The model under review builds one solid part; all positions refer to its coordinate system, in mm. Face numbers are marked on the shaded views. Round coordinates to 2 decimals unless told otherwise and drop trailing zeros. Order: outer loops, then holes, each group sorted by start corner. A loop starts at its lowest first (then second) coordinate and runs counter-clockwise, first axis right, second up. Notation, with made-up numbers: M 89,36.25 L 143,36.25 A20 ccw 143,49.25 Z; hole C -16.5,-33.5 d10. An arc over 180 degrees is marked long. Answer as a JSON object with one key per item and string values. Group by question number.
1) Consider section B-B, the plane z = -2.5. Write out the cut boundary in (x, y).
2) The part is to be moulded in two halves that separate along X. For the marked faces 1 and 2, say which applies: +X half, -X half, draft (parallel to the pull), parting line (faces both ways), or undercut.
3) Consider section A-A, the plane x = 5. Write out the cut boundary in (y, z), then the cut area to 3 significant figures.
4) To check wall thickness, follow line 1 (Y direction, x = -85, z = 0.1); line 2 (X direction, y = 121.75, z = 0.4); line 3 (X direction, y = 29, z = -4.75). State the ranges of each line that lie inside material, in increasing order.
5) Insertion check: pin 1 Ø6 at (x, y) = (5.5, 46.5) entering from -Z; pin 2 Ø3 at (x, y) = (5, 31.75) entering from -Z; pin 3 Ø3.5 at (y, z) = (56, -2) entering from -X; pin 4 Ø1 at (y, z) = (90.5, -2) entering from +X. Each pin has a flat end and moves straight along its axis. Give the tip position at first contact, or say it passes through.
6) Consider section D-D, the plane y = 89.5. Write out the cut boundary in (x, z), then the cut area to 3 significant figures.
7) Consider section C-C, the plane y = 121.75. Write out the cut boundary in (x, z).
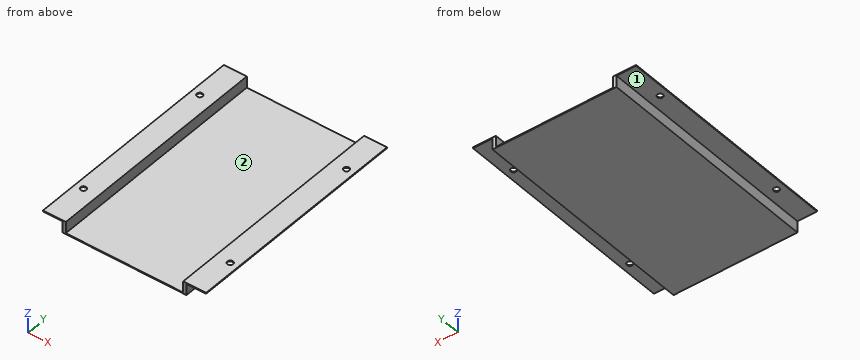
Autodesk Inventor part; units mm, degrees
ref_plane "YZ Plane" through (0, 0, 0) normal (1, 0, 0) x (0, 1, 0)
ref_plane "XZ Plane" through (0, 0, 0) normal (0, 1, 0) x (-1, 0, 0)
ref_plane "XY Plane" through (0, 0, 0) normal (0, 0, 1) x (1, 0, 0)
sketch "Skizze1" plane through (0, 0, 0) normal (0, 0, 1) x (1, 0, 0)
  line L0 (-90, 0) -> (-90, 36.75) construction
  line L1 (10, 0) -> (10, 36.75) construction
  line L2 (-90, 116.75) -> (-90, 147.085) construction
  line L3 (10, 147.085) -> (10, 116.75) construction
  circle A0 centre (-85, 121.75) radius 1.75
  circle A1 centre (5, 121.75) radius 1.75
  circle A2 centre (-85, 31.75) radius 1.75
  circle A3 centre (5, 31.75) radius 1.75
  line L4 (-90, 6.75) -> (10, 6.75)
  line L5 (10, 6.75) -> (10, 146.75)
  line L6 (10, 146.75) -> (-90, 146.75)
  line L7 (-90, 146.75) -> (-90, 6.75)
  point P0 (0, 0)
  dimension "d0" = 25
  dimension "d1" = 25
extrude "Extrusion1" add sketch "Skizze1" along normal blind 0.6
sketch "Skizze2" plane through (0, 0, 0) normal (0, 0, -1) x (-1, 0, 0)
  line L0 (90, 6.75) -> (-10, 6.75)
  line L1 (-10, 146.75) -> (90, 146.75)
  line L2 (2, 6.75) -> (78, 6.75)
  line L3 (78, 6.75) -> (78, 146.75)
  line L4 (78, 146.75) -> (2, 146.75)
  line L5 (2, 146.75) -> (2, 6.75)
  line L6 (-10, 6.75) -> (-10, 146.75)
  line L7 (90, 146.75) -> (90, 6.75)
  line L8 (78, 146.75) -> (2, 146.75)
  line L9 (2, 146.75) -> (2, 6.75)
  line L10 (2, 6.75) -> (78, 6.75)
  line L11 (78, 6.75) -> (78, 146.75)
  point P0 (0, 0)
  dimension "d4" = 12
  dimension "d5" = 12
extrude "Extrusion3" add sketch "Skizze2" along normal blind 7 contours L0 L5 L1 L3
sketch "Skizze3" plane through (0, 0, 0.6) normal (0, 0, 1) x (1, 0, 0)
  line L0 (-2, 6.75) -> (-78, 6.75) construction
  line L1 (-78, 6.75) -> (-78, 146.75) construction
  line L2 (-78, 146.75) -> (-2, 146.75) construction
  line L3 (-2, 146.75) -> (-2, 6.75) construction
  line L4 (-90, 6.75) -> (10, 6.75)
  line L5 (-78, 146.75) -> (-2, 146.75)
  line L6 (-4, 6.75) -> (-76, 6.75)
  line L7 (-76, 6.75) -> (-76, 146.75)
  line L8 (-76, 146.75) -> (-4, 146.75)
  line L9 (-4, 146.75) -> (-4, 6.75)
  point P0 (0, 0)
  dimension "d10" = 2
  dimension "d11" = 2
extrude "Extrusion4" cut sketch "Skizze3" against normal blind 7
properties part number "PCB-Mount"
Results list:
{
 "1": {"outline": "M -78,6.75 L -76,6.75 L -76,146.75 L -78,146.75 Z; M -4,6.75 L -2,6.75 L -2,146.75 L -4,146.75 Z"},
 "2": {"face 1": "draft", "face 2": "undercut"},
 "3": {"outline": "M 6.75,0 L 30,0 L 30,0.6 L 6.75,0.6 Z; M 33.5,0 L 120,0 L 120,0.6 L 33.5,0.6 Z; M 123.5,0 L 146.75,0 L 146.75,0.6 L 123.5,0.6 Z", "area": "79.8 mm^2"},
 "4": {"line 1": "6.75 to 30, 33.5 to 120, 123.5 to 146.75", "line 2": "-90 to -86.75, -83.25 to -76, -4 to 3.25, 6.75 to 10", "line 3": "-78 to -76, -4 to -2"},
 "5": {"pin 1": "z = 0", "pin 2": "through", "pin 3": "x = -78", "pin 4": "x = -2"},
 "6": {"outline": "M -90,0 L -78,0 L -78,-7 L -2,-7 L -2,0 L 10,0 L 10,0.6 L -4,0.6 L -4,-6.4 L -76,-6.4 L -76,0.6 L -90,0.6 Z", "area": "88.0 mm^2"},
 "7": {"outline": "M -90,0 L -86.75,0 L -86.75,0.6 L -90,0.6 Z; M -83.25,0 L -78,0 L -78,-7 L -2,-7 L -2,0 L 3.25,0 L 3.25,0.6 L -4,0.6 L -4,-6.4 L -76,-6.4 L -76,0.6 L -83.25,0.6 Z; M 6.75,0 L 10,0 L 10,0.6 L 6.75,0.6 Z"}
}
